The drawing under review shows one solid part. Ordinate dimensions are in mm from its lowest x, y, z. Give positions to 0.01 mm unless a question says otherwise; leave off trailing zeros. Order: outer loops, then holes, each group sorted by start corner. A loop starts at its lowest first (then second) coordinate and runs counter-clockwise, first axis right, second up. Notation, with made-up numbers: (60.25, 6.5) - (87.25, 6.5) arc R32 ccw to (87.25, 40.5) - close; hole circle Ø7 at (45.25, 34.5). An arc over 180 degrees is marked (long way). Answer as a JSON object with one key per item and string values. Group by question number.
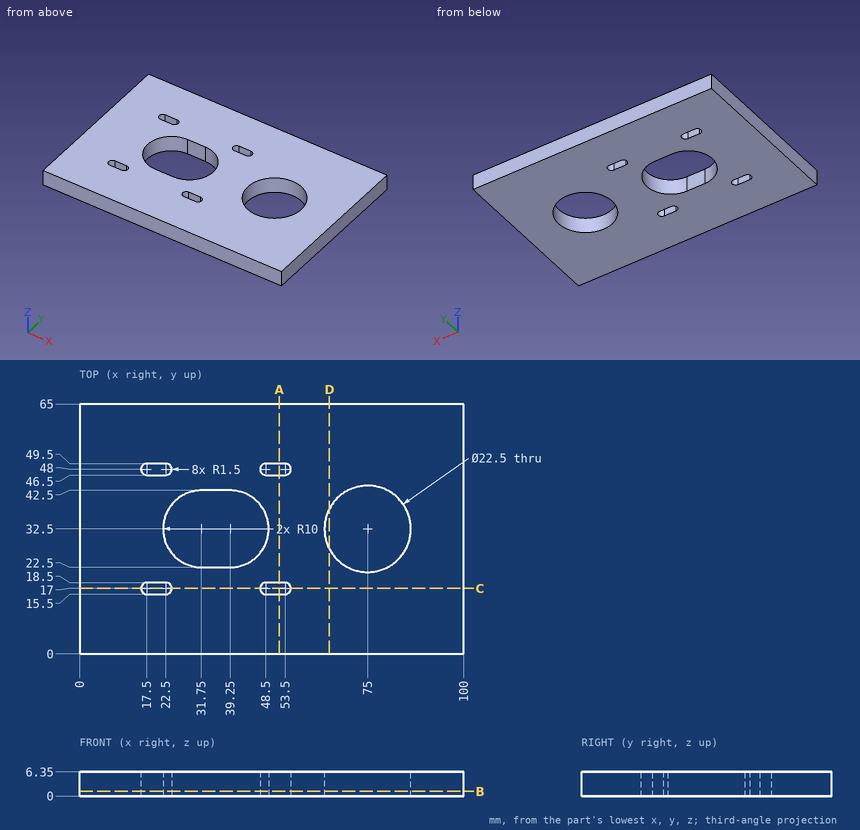
1) Consider section D-D (x = 65). Give the boundary of the cut face in (y, z), plus the area to 3 significant figures.
2) Consider section C-C (y = 17). Give the boundary of the cut face in (x, z), plus the area to 3 significant figures.
3) For line 1 (Y direction, x = 75, z = 3.5); line 2 (Y direction, x = 21.5, z = 2.25); line 3 (X direction, y = 24, z = 0.75), list the stretches that pass through material, from the lowest coordinate up.
4) Consider section B-B (z = 1.25). Give the boundary of the cut face in (x, y).
5) Consider section A-A (x = 52). Give the boundary of the cut face in (y, z).
Result set:
{
 "1": {"outline": "(0, 0) - (27.35, 0) - (27.35, 6.35) - (0, 6.35) - close; (37.65, 0) - (65, 0) - (65, 6.35) - (37.65, 6.35) - close", "area": "347 mm2"},
 "2": {"outline": "(0, 0) - (16, 0) - (16, 6.35) - (0, 6.35) - close; (24, 0) - (47, 0) - (47, 6.35) - (24, 6.35) - close; (55, 0) - (100, 0) - (100, 6.35) - (55, 6.35) - close", "area": "533 mm2"},
 "3": {"line 1": "y = 0 to 21.25, 43.75 to 65", "line 2": "y = 0 to 15.5, 18.5 to 46.5, 49.5 to 65", "line 3": "x = 0 to 26.48, 44.52 to 67.63, 82.37 to 100"},
 "4": {"outline": "(0, 0) - (100, 0) - (100, 65) - (0, 65) - close; hole (17.5, 15.5) - (22.5, 15.5) arc R1.5 ccw to (22.5, 18.5) - (17.5, 18.5) arc R1.5 ccw to start; hole (17.5, 46.5) - (22.5, 46.5) arc R1.5 ccw to (22.5, 49.5) - (17.5, 49.5) arc R1.5 ccw to start; hole (31.75, 22.5) - (39.25, 22.5) arc R10 ccw to (39.25, 42.5) - (31.75, 42.5) arc R10 ccw to start; hole (48.5, 15.5) - (53.5, 15.5) arc R1.5 ccw to (53.5, 18.5) - (48.5, 18.5) arc R1.5 ccw to start; hole (48.5, 46.5) - (53.5, 46.5) arc R1.5 ccw to (53.5, 49.5) - (48.5, 49.5) arc R1.5 ccw to start; hole circle Ø22.5 at (75, 32.5)"},
 "5": {"outline": "(0, 0) - (15.5, 0) - (15.5, 6.35) - (0, 6.35) - close; (18.5, 0) - (46.5, 0) - (46.5, 6.35) - (18.5, 6.35) - close; (49.5, 0) - (65, 0) - (65, 6.35) - (49.5, 6.35) - close"}
}
